Verification items for the finished model (mm, model axes). A direction names the side the tool comes from. Give positions to 0.01 mm unless a question says otherwise; leave off trailing zeros. Loops run counter-clockwise (first coordinate to the right, second up) from the corner with the lowest first, then second, coordinate; pieces in that order, holes last. Notation, with made-up numbers: (-32, -17.5) - (-5, -17.5) arc R33 ccw to (-5, 14.5) - close; hole circle Ø2 at (29, 74). An arc over 180 degrees is marked (long way). One line per item, written item: value. Start each with the question number.
1. Access from +Z, -Z, +X, -X, +Y, -Y to the whole of each face (thin tool, end or side, straight path). Record for faces 5 (the cylindrical face through (-2.685, -0.01, 0.596)), 6 (the cylindrical face through (-2, 0, 0)).
2. Gauge pin test, flat ends, axial feed: pin 1 (2 mm diameter, centred on x = 1.5, z = -3.5, fed in from +Y); pin 2 (1.5 mm diameter, centred on x = 5, y = -1, fed in from -Z). Record the tip position at first contact, or that the pin passes through.
3. Sectioned sample at C-C (y = -0.55). Record the cut outline in (x, z).
4. Sectioned sample at B-B (z = 0). Record the cut outline in (x, y), plus the area to 3 significant figures.
5. Scan lines: L1, parallel to X at y = -0.6, z = 0; L2, parallel to X at y = 0.9, z = 0; L3, parallel to Y at x = 3.75, z = -3.5. Record each from-to range of solid material in increasing order. Write a range as [from, to].
6. Sectioned sample at A-A (x = 0). Record the cut outline in (y, z).
7. Sectioned sample at D-D (x = 3.5). Record the cut outline in (y, z), plus the area to 3 significant figures.
8. Mould release check, pull along Y, two halves, no side actions. Record for faces 1 (the flat face through (-2, 2.5, 1)), 2 (the flat face through (-3, -0.75, 0)), 3 (the flat face through (-2, -2.5, -1)), 4 (the flat face through (-3, 0.75, 0)): pulls with the +Y half, pulls with the -Y half, needs draft (parallel to the pull), parting line crosses it, or undercut.
from build123d import *


with BuildPart() as part:
    # 草图2 → 旋转1 (revolve)
    with BuildSketch(Plane(origin=(0, 0, 0), x_dir=(0, 0, -1), z_dir=(1, 0, 0))):
        with BuildLine():
            Line((6.463548925, 0.75), (2.75, 0.75))
            Line((2.75, 0.75), (2.75, -0.75))
            Line((2.75, -0.75), (6.463548925, -0.75))
            ThreePointArc((6.463548925, -0.75), (4.689135949, -1.799773377), (2.75, -2.5))
            Line((2.75, -2.5), (2, -2.5))
            Line((2, -2.5), (2, 2.5))
            Line((2, 2.5), (2.75, 2.5))
            ThreePointArc((2.75, 2.5), (4.689135949, 1.799773377), (6.463548925, 0.75))
        make_face()
    revolve(axis=Axis((0, 32.338552752, 0), (0, -1, 0)))


solid = part.part
Results are:
1. face 5: none
1. face 6: +Y, -Y
2. pin 1: stops at y = 2.48
2. pin 2: stops at z = -4.83
3. outline: circle Ø5.5 at (0, 0); hole circle Ø4 at (0, 0)
4. outline: (-6.46, -0.75) arc R11 ccw to (-2.75, -2.5) - (-2, -2.5) - (-2, 2.5) - (-2.75, 2.5) arc R11 ccw to (-6.46, 0.75) - (-2.75, 0.75) - (-2.75, -0.75) - close; (2, -2.5) - (2.75, -2.5) arc R11 ccw to (6.46, -0.75) - (2.75, -0.75) - (2.75, 0.75) - (6.46, 0.75) arc R11 ccw to (2.75, 2.5) - (2, 2.5) - close
4. area: 22.6 mm^2
5. L1: x = [-2.75, -2], [2, 2.75]
5. L2: x = [-6.25, -2], [2, 6.25]
5. L3: y = [-1.58, -0.75], [0.75, 1.58]
6. outline: (-2.5, -2.75) arc R11 ccw to (-0.75, -6.46) - (-0.75, -2.75) - (0.75, -2.75) - (0.75, -6.46) arc R11 ccw to (2.5, -2.75) - (2.5, -2) - (-2.5, -2) - close; (-2.5, 2) - (2.5, 2) - (2.5, 2.75) arc R11 ccw to (0.75, 6.46) - (0.75, 2.75) - (-0.75, 2.75) - (-0.75, 6.46) arc R11 ccw to (-2.5, 2.75) - close
7. outline: (-0.75, -5.43) - (-0.75, 5.43) arc R10.43 ccw to start; (0.75, -5.43) arc R10.43 ccw to (0.75, 5.43) - close
7. area: 22.5 mm^2
8. face 1: pulls with the +Y half
8. face 2: undercut
8. face 3: pulls with the -Y half
8. face 4: undercut
